from build123d import *

# Parameters (mm, degrees)
F1_DEPTH = 12.7
F2_R     = 1.867032
F3_DEPTH = 14.478


with BuildPart() as f1:
    # F0 (on Front) → F1 (new body)
    with BuildSketch(Plane.XZ):
        Polygon((-0.699146, 29.252446), (-25.682935, 14.020745), (-24.983788, -15.231702), (0.699146, -29.252446), (25.682935, -14.020745), (24.983788, 15.231702), align=None)
    extrude(amount=F1_DEPTH)

    # F2 (on face) → F3 (cut)
    with BuildSketch(Plane.XZ.offset(12.7)):
        with Locations((-22.552457, 10.605652)):
            Circle(F2_R)
        with Locations((-19.917389, -11.265242)):
            Circle(F2_R)
        with Locations((-3.322549, -24.042027)):
            Circle(F2_R)
        with Locations((-4.203008, -8.466095)):
            Circle(F2_R)
        with Locations((9.971874, 2.4621)):
            Circle(F2_R)
        with Locations((22.114325, -11.681865)):
            Circle(F2_R)
        with Locations((21.476673, -5.378575)):
            Circle(F2_R)
        with Locations((22.459481, 0)):
            Circle(F2_R)
        with Locations((22.506732, 5.011312)):
            Circle(F2_R)
        with Locations((19.734677, 12.446447)):
            Circle(F2_R)
        with Locations((-0.272807, 24.720894)):
            Circle(F2_R)
        with Locations((-9.246618, 20.632951)):
            Circle(F2_R)
        with Locations((-9.246618, 15.130831)):
            Circle(F2_R)
        with Locations((-10.316476, 9.475874)):
            Circle(F2_R)
        with Locations((-8.940945, 4.432264)):
            Circle(F2_R)
        with Locations((-9.399456, -1.222693)):
            Circle(F2_R)
        with Locations((-9.399456, -6.571977)):
            Circle(F2_R)
        with Locations((-9.705129, -12.074097)):
            Circle(F2_R)
        with Locations((-10.163639, -16.812034)):
            Circle(F2_R)
        with Locations((-15.66576, -14.672321)):
            Circle(F2_R)
        with Locations((-14.137393, -7.030488)):
            Circle(F2_R)
        with Locations((-13.373209, -2.445387)):
            Circle(F2_R)
        with Locations((-14.290229, 4.126591)):
            Circle(F2_R)
        with Locations((-14.290229, 9.934384)):
            Circle(F2_R)
        with Locations((-13.526046, 15.742177)):
            Circle(F2_R)
        with Locations((-18.111147, 12.685444)):
            Circle(F2_R)
        with Locations((-21.779226, 4.737937)):
            Circle(F2_R)
        with Locations((-18.569656, 0.152837)):
            Circle(F2_R)
        with Locations((-19.79235, -5.50212)):
            Circle(F2_R)
        with Locations((-22.237737, -1.681203)):
            Circle(F2_R)
        with Locations((-5.120028, 19.257421)):
            Circle(F2_R)
        with Locations((-4.661518, 14.213812)):
            Circle(F2_R)
        with Locations((-3.897335, 9.323037)):
            Circle(F2_R)
        with Locations((-1.299111, 5.96063)):
            Circle(F2_R)
        with Locations((4.967192, 3.973754)):
            Circle(F2_R)
        with Locations((14.595903, 3.056734)):
            Circle(F2_R)
        with Locations((17.805472, 7.641834)):
            Circle(F2_R)
        with Locations((13.373209, 12.074097)):
            Circle(F2_R)
        with Locations((9.093783, 15.130831)):
            Circle(F2_R)
        with Locations((4.967192, 18.798912)):
            Circle(F2_R)
        with Locations((0.534929, 18.034728)):
            Circle(F2_R)
        with Locations((1.299111, 13.908138)):
            Circle(F2_R)
        with Locations((8.482436, 8.558854)):
            Circle(F2_R)
        with Locations((-3.897335, 1.681203)):
            Circle(F2_R)
        with Locations((-4.355845, -3.362407)):
            Circle(F2_R)
        with Locations((-3.744498, -13.143954)):
            Circle(F2_R)
        with Locations((-4.203008, -19.257421)):
            Circle(F2_R)
        with Locations((0.687765, -20.785788)):
            Circle(F2_R)
        with Locations((6.648396, -21.244299)):
            Circle(F2_R)
        with Locations((14.901575, -15.436505)):
            Circle(F2_R)
        with Locations((18.111147, -9.781547)):
            Circle(F2_R)
        with Locations((16.124269, -1.83404)):
            Circle(F2_R)
        with Locations((6.342723, -1.83404)):
            Circle(F2_R)
        with Locations((2.216131, -4.279427)):
            Circle(F2_R)
        with Locations((1.604785, -10.698567)):
            Circle(F2_R)
        with Locations((3.285989, -15.895015)):
            Circle(F2_R)
        with Locations((8.482436, -16.506363)):
            Circle(F2_R)
        with Locations((11.99768, -10.698567)):
            Circle(F2_R)
        with Locations((6.495558, -10.392894)):
            Circle(F2_R)
        with Locations((13.373209, -6.724814)):
            Circle(F2_R)
    extrude(amount=-F3_DEPTH, mode=Mode.SUBTRACT)


solid = f1.part
Geometry: final body of the model. Coordinates: model frame, mm. Coordinates: 2 decimals unless noted, no trailing zeros. Put each result on its own line as item: value. Start each with the question number.
Q1. Pull-direction query (Z, two-part tool) for faces 1 (the flat face through (12.322, -6.261, 22.144)), 2 (the cylindrical face through (18.36, -6.44, 13.71)), 3 (the flat face through (0, 0, -6)); classes: released by +Z, released by -Z, zero draft, split by the parting line, or undercut.
Q2. Line query: line 1 (Z direction, x = 23, y = -5.5); line 2 (X direction, y = -11.5, z = 15.5); line 3 (Z direction, x = 9.5, y = -6.5). Output: solid intervals per line, ascending.
Q3. Cut plane A-A, the plane y = -4.75. Give the number of separate pieces and of enclosed holes in the cut face, and give its area (3 significant figures).
Q4. Pin query (flat end, axial travel): pin 1 Ø5 at (x, y) = (-12, -6) entering from +Z; pin 2 Ø6 at (y, z) = (-9.5, 8) entering from -X; pin 3 Ø1 at (x, y) = (-6, -8.5) entering from -Z. Return the tip coordinate at first contact, or that it passes through.
Filled sheet:
1. face 1: released by +Z
1. face 2: undercut
1. face 3: zero draft
2. line 1: -15.66 to -13.33, -10.04 to -6.46, -4.3 to -1.79, 1.79 to 3.21, 6.81 to 16.31
2. line 2: -23.26 to -15.38, -11.67 to -11.08, -7.42 to -6.01, -3.31 to 0.32, 2.27 to 7.26, 10.92 to 24.49
2. line 3: -23.89 to -18.07, -14.94 to 0.66, 4.27 to 6.99, 10.12 to 13.31, 16.95 to 23.68
3. separate pieces: 1
3. enclosed holes: 60
3. area: 1,570 mm²
4. pin 1: z = 23.89
4. pin 2: x = -25.61
4. pin 3: z = -25.87
